Check sheet for the modelled part. Datum: model origin and axes. Units: mm. Face numbers are marked on the shaded views. A direction names the side the tool comes from. Round coordinates to 2 decimals unless told otherwise and drop trailing zeros. Order: outer loops, then holes, each group sorted by start corner. A loop starts at its lowest first (then second) coordinate and runs counter-clockwise, first axis right, second up. Notation, with made-up numbers: (51.25, 79.5) -> (89.25, 79.5) arc R37 cw to (89.25, 116.5) -> close; hole circle Ø1 at (68, 69). An arc over 180 degrees is marked (long way). Answer in a Markdown table with one row per item.
```python
from build123d import *

# Parameters (mm, degrees)
SZKIC1_R                    = 10.3
DODANIE_WYCI_GNI_CIE1_DEPTH = 35.75
OTWORY_USTALAJ_CE_2_5MM2_D  = 2.25
DODANIE_WYCI_GNI_CIE3_START = -7
DODANIE_WYCI_GNI_CIE3_DEPTH = 7
OTWORY_USTALAJ_CE_2_5MM3_D  = 22
SZKIC12_R                   = 0.7
WYTNIJ_WYCI_GNI_CIE1_DEPTH  = 7


with BuildPart() as part:
    # Szkic1 → Dodanie-wyci_gni_cie1 (new body)
    with BuildSketch(Plane(origin=(0, 0, 0), x_dir=(1, 0, 0), z_dir=(0, 1, 0))):
        with Locations(Location((0, 0, 0), (0, 0, 270))):
            Circle(SZKIC1_R)
    extrude(amount=DODANIE_WYCI_GNI_CIE1_DEPTH)

    # Otwory ustalaj_ce _2.5mm2 (through all)
    with Locations(Plane.XZ):
        with Locations((0, 0)):
            Hole(OTWORY_USTALAJ_CE_2_5MM2_D / 2)

    # Szkic7 → Dodanie-wyci_gni_cie3 (add)
    with BuildSketch(Plane(origin=(0, 35.75, 0), x_dir=(1, 0, 0), z_dir=(0, 1, 0)).offset(DODANIE_WYCI_GNI_CIE3_START)):
        with BuildLine():
            Line((66.943357066, 13.440701035), (0, 10.3))
            ThreePointArc((0, 10.3), (10.077130906, 2.131063748), (4.169904535, -9.418168408))
            add(Edge.make_bspline(
                [(4.169904535, -9.418168408), (22.461776037, -3.24596138), (41.934151815, -4.077243057), (61.820006497, -11.893378905)],
                knots=[0, 0, 0, 0, 1, 1, 1, 1], degree=3))
            ThreePointArc((61.820006497, -11.893378905), (81.439431711, -2.675954354), (66.943357066, 13.440701035))
        make_face()
    extrude(amount=DODANIE_WYCI_GNI_CIE3_DEPTH)

    # Otwory ustalaj_ce _2.5mm3 (through all)
    with Locations(Plane(origin=(0, 35.75, 0), x_dir=(1, 0, 0), z_dir=(0, 1, 0))):
        with Locations((68.207301561, 0)):
            Hole(OTWORY_USTALAJ_CE_2_5MM3_D / 2)

    # Szkic12 → Wytnij-wyci_gni_cie1 (cut)
    with BuildSketch(Plane.XZ):
        with Locations(Location((7.24, 0, 0), (0, 0, 270))):
            Circle(SZKIC12_R)
        with Locations(Location((-7.24, 0, 0), (0, 0, 270))):
            Circle(SZKIC12_R)
        with Locations(Location((0, -7.24, 0), (0, 0, 270))):
            Circle(SZKIC12_R)
        with Locations(Location((0, 7.24, 0), (0, 0, 270))):
            Circle(SZKIC12_R)
    extrude(amount=-WYTNIJ_WYCI_GNI_CIE1_DEPTH, mode=Mode.SUBTRACT)


solid = part.part
```
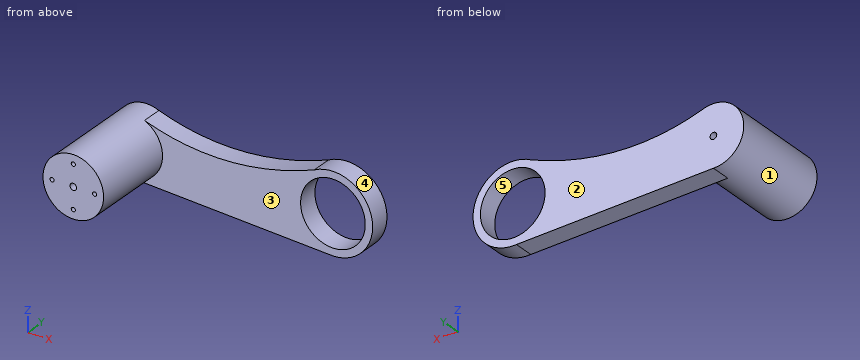
(1) Depth check by flat-ended pin: pin 1 Ø0.7 at (x, z) = (7, 0) entering from -Y; pin 2 Ø5 at (x, y) = (28, 31) entering from +Z; pin 3 Ø10 at (y, z) = (27.5, 6.5) entering from -X. Enter the tip coordinate at first touch or a pass-through.
Solutions:
| item | result |
|---|---|
| pin 1 | y = 7 |
| pin 2 | z = 5.41 |
| pin 3 | x = -10.19 |
(2) Section check D-D on y = 30.5. Give the number of separate pieces and of enclosed holes in the cut face, plus the area to 3 significant figures.
Solutions:
| item | result |
|---|---|
| separate pieces | 1 |
| enclosed holes | 2 |
| area | 1,420 mm^2 |
(3) Section check A-A on z = -4.25. Record the boundary of the cut face in (x, y).
Solutions:
| item | result |
|---|---|
| outline | (-9.38, 0) -> (9.38, 0) -> (9.38, 28.75) -> (58.06, 28.75) -> (58.06, 35.75) -> (-9.38, 35.75) -> close; (78.35, 28.75) -> (81.02, 28.75) -> (81.02, 35.75) -> (78.35, 35.75) -> close |
(4) Section check B-B on x = 63. Record the boundary of the cut face in (y, z).
Solutions:
| item | result |
|---|---|
| outline | (28.75, -13.26) -> (35.75, -13.26) -> (35.75, -9.69) -> (28.75, -9.69) -> close; (28.75, 9.69) -> (35.75, 9.69) -> (35.75, 12.46) -> (28.75, 12.46) -> close |
(5) Scan lines: probe 1 along X at (y, z) = (34.5, 0.25); probe 2 along Y at (x, z) = (18.5, -6.25); probe 3 along X at (y, z) = (5.25, -7.24). Record each from-to range of solid material in increasing order. Write a range as from..to.
Solutions:
| item | result |
|---|---|
| probe 1 | -10.3..-1.1, 1.1..57.21, 79.2..81.7 |
| probe 2 | 28.75..35.75 |
| probe 3 | -7.33..-0.7, 0.7..7.33 |
(6) Tool access check on the marked faces 1 and 2. Record the directions out of +Z, -Z, +X, -X, +Y, -Y that give a thin tool (end or side, any length) a straight path to the whole face; none if there is none.
Solutions:
| item | result |
|---|---|
| face 1 | -Y |
| face 2 | +Z, -Z, +X, -X, +Y |
(7) Section check C-C on y = 13. Record the boundary of the cut face in (x, z) (3 decimals).
Solutions:
| item | result |
|---|---|
| outline | circle Ø20.6 at (0, 0); hole circle Ø2.25 at (0, 0) |
(8) Draft check along Z on the marked faces 3, 4 and 5. Enter one of: pulls with the +Z half, pulls with the -Z half, needs draft (parallel to the pull), parting line crosses it, or undercut.
Solutions:
| item | result |
|---|---|
| face 3 | needs draft |
| face 4 | parting line crosses it |
| face 5 | undercut |
